Here's how the part is built. I have some questions about the finished solid (model axes, mm). Round coordinates to 2 decimals unless told otherwise and drop trailing zeros. Order: outer loops, then holes, each group sorted by start corner. A loop starts at its lowest first (then second) coordinate and runs counter-clockwise, first axis right, second up. Notation, with made-up numbers: M 69,79 L 102,79 A13 ccw 102,88 Z; hole C 48,68.25 d9. An arc over 180 degrees is marked long. Answer as CSV lines item,"result". Start each with the question number.
```python
from build123d import *

# Parameters (mm, degrees)
BOSS_EXTRUDE1_DEPTH      = 5
BOSS_EXTRUDE1_DEPTH_BACK = 5
SKETCH3_R                = 1.2
CUT_EXTRUDE1_DEPTH       = 10
SKETCH4_W                = 13.374580466
SKETCH4_H                = 4.798064452
CUT_EXTRUDE2_DEPTH       = 0.2
CUT_EXTRUDE3_DEPTH       = 10


with BuildPart() as part:
    # Sketch2 → Boss-Extrude1 (new, two sides: drawn at the far end of the back side and taken through both)
    with BuildSketch(Plane(origin=(0, 0, 0), x_dir=(1, 0, 0), z_dir=(0, 1, 0)).offset(-BOSS_EXTRUDE1_DEPTH_BACK)):
        with BuildLine():
            Line((0, 2.2), (10, 2.2))
            Line((10, 2.2), (10, -2.2))
            Line((10, -2.2), (0, -2.2))
            ThreePointArc((0, -2.2), (-2.2, 0), (0, 2.2))
        make_face()
    extrude(amount=BOSS_EXTRUDE1_DEPTH + BOSS_EXTRUDE1_DEPTH_BACK)

    # Sketch3 → Cut-Extrude1 (cut)
    with BuildSketch(Plane(origin=(0, 5, 0), x_dir=(1, 0, 0), z_dir=(0, 1, 0))):
        with Locations(Location((0, 0, 0), (0, 0, 270))):
            Circle(SKETCH3_R)
    extrude(amount=-CUT_EXTRUDE1_DEPTH, mode=Mode.SUBTRACT)

    # Sketch4 → Cut-Extrude2 (cut)
    with BuildSketch(Plane.XZ.offset(5)):
        with Locations((3.312709767, -0.199032226)):
            Rectangle(SKETCH4_W, SKETCH4_H)
    cut_extrude2 = extrude(amount=-CUT_EXTRUDE2_DEPTH, mode=Mode.SUBTRACT)

    # Mirror1: Cut-Extrude2 across plane
    add(cut_extrude2.mirror(Plane.ZX), mode=Mode.SUBTRACT)

    # Sketch5 → Cut-Extrude3 (cut)
    with BuildSketch(Plane(origin=(0, 4.8, 0), x_dir=(1, 0, 0), z_dir=(0, 1, 0))):
        Polygon((2.645324972, -2.2), (10, 0), (10, -2.2), align=None)
    extrude(amount=-CUT_EXTRUDE3_DEPTH, mode=Mode.SUBTRACT)


solid = part.part
```
Item 1: For P1, Ø1.4, axis at x = 0, z = 0, coming from the +Y side, with a flat end and sliding along its axis, tell me the tip position at first contact or that it passes through.
Item 2: If I drill on line 1 along X through (y, z) = (-2.75, -0.5); line 2 along Z through (x, y) = (0.5, -3); line 3 along X through (y, z) = (-0.25, -0.4), over which ranges is the centre line in solid material (lowest first)?
Item 3: If we section it at A-A on z = -0.7: Please give me the cut outline in (x, y).
Item 4: If we section it at C-C on x = -0.75: Please give me the cut outline in (y, z).
Item 5: We'd pull the mould along Z, two halves only. Please class faces 1 (the cylindrical face through (1.01, 0.07, 0.65)), 2 (the flat face through (1, 0, 2.2)), 3 (the flat face through (4, 4.8, 0)): pulls with the +Z half, pulls with the -Z half, needs draft (parallel to the pull), parting line crosses it, or undercut.
Item 6: If we section it at B-B on y = 2.25: Please give me the cut outline in (x, z).
Item 7: If we section it at D-D on x = 8.75: Please give me the cut outline in (y, z), and give its area (3 significant figures).
Geometry says:
1,P1,"through"
2,line 1,"-2.14 to -1.09, 1.09 to 10"
2,line 2,"-2.2 to -1.09, 1.09 to 2.2"
2,line 3,"-2.16 to -1.13, 1.13 to 10"
3,outline,"M -2.09,-4.8 L -0.97,-4.8 L -0.97,4.8 L -2.09,4.8 Z; M 0.97,-4.8 L 10,-4.8 L 10,4.8 L 0.97,4.8 Z"
4,outline,"M -4.8,-2.07 L 4.8,-2.07 L 4.8,-0.94 L -4.8,-0.94 Z; M -4.8,0.94 L 4.8,0.94 L 4.8,2.07 L -4.8,2.07 Z"
5,face 1,"undercut"
5,face 2,"pulls with the +Z half"
5,face 3,"needs draft"
6,outline,"M 0,-2.2 L 10,-2.2 L 10,0 L 2.65,2.2 L 0,2.2 A2.2 ccw Z; hole C 0,0 d2.4"
7,outline,"M -4.8,-2.2 L 4.8,-2.2 L 4.8,0.37 L -4.8,0.37 Z"
7,area,"24.7 mm²"
